Answer from the drawing. Dimensions are ordinates in mm from the lowest x, y and z of the part. Round coordinates to 2 decimals unless told otherwise and drop trailing zeros. Order: outer loops, then holes, each group sorted by start corner. A loop starts at its lowest first (then second) coordinate and runs counter-clockwise, first axis right, second up. Notation, with made-up numbers: M 1.25,-33.5 L 42.25,-33.5 A20 cw 42.25,-16.5 Z; hole C 6,-37.5 d9. An arc over 180 degrees is marked long. Use one line per item in the form item = value. Start each with the question number.
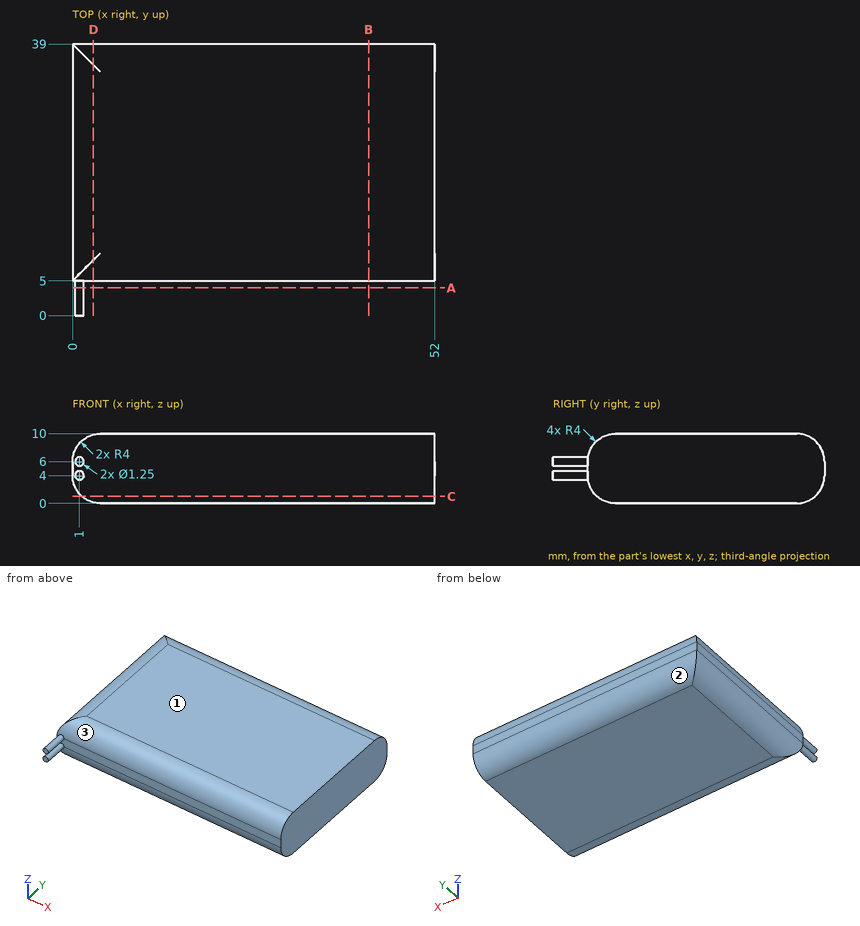
Item 1: Section C-C (z = 1) is taken. Write down the section's boundary in (x, y), and give its area (3 significant figures).
Item 2: Section D-D (x = 3) is taken. Write down the section's boundary in (y, z), and give its area (3 significant figures).
Item 3: Given P1, Ø0.6, axis at x = 21, z = 5, coming from the -Y side; P2, Ø2, axis at x = 21.5, z = 9, coming from the +Y side, each flat-ended and moving along its own axis, determine where each tip first touches the part or whether it passes through.
Item 4: Section B-B (x = 42.5) is taken. Write down the section's boundary in (y, z), and give its area (3 significant figures).
Item 5: For a pull along Y with two mould halves and no side action, classify the marked faces 1, 2 and 3 as pulls with the +Y half, pulls with the -Y half, needs draft (parallel to the pull), parting line crosses it, or undercut.
Item 6: Section A-A (y = 4) is taken. Write down the section's boundary in (x, z) (3 decimals), and give its area (3 significant figures).
Item 7: Find the intervals of material crossed by L1, parallel to Y at x = 16.5, z = 5; L2, parallel to X at y = 36, z = 7; L3, parallel to Z at x = 43, y = 7, in increasing order. Write a range as [from, to].
The answers:
q1.outline = M 1.35,6.35 L 52,6.35 L 52,37.65 L 1.35,37.65 Z
q1.area = 1,580 mm²
q2.outline = M 5,4 A4 ccw 8,0.13 L 36,0.13 A4 ccw 39,4 L 39,6 A4 ccw 36,9.87 L 8,9.87 A4 ccw 5,6 Z
q2.area = 319 mm²
q3.P1 = 5
q3.P2 = 38.46
q4.outline = M 5,4 A4 ccw 9,0 L 35,0 A4 ccw 39,4 L 39,6 A4 ccw 35,10 L 9,10 A4 ccw 5,6 Z
q4.area = 326 mm²
q5.face_1 = needs draft
q5.face_2 = pulls with the +Y half
q5.face_3 = pulls with the -Y half
q6.outline = C 1,4 d1.25; C 1,6 d1.25
q6.area = 2.45 mm²
q7.L1 = [5, 39]
q7.L2 = [0.13, 52]
q7.L3 = [0.54, 9.46]
